Work out the finished part from the listing and answer in its coordinate system (mm). A direction names the side the tool comes from. Round coordinates to 2 decimals unless told otherwise and drop trailing zeros. Order: outer loops, then holes, each group sorted by start corner. A loop starts at its lowest first (then second) coordinate and runs counter-clockwise, first axis right, second up. Notation, with made-up numbers: M -21.5,54.25 L 14.5,54.25 A25 cw 14.5,89.25 Z; hole C -17,4 d1. An arc over 180 degrees is marked long. Return JSON: item names as keys, results as strings.
from build123d import *

# Parameters (mm, degrees)
SKETCH1_W           = 23
SKETCH1_H           = 30
SKETCH1_R           = 2.5
BOSS_EXTRUDE1_DEPTH = 6
BOSS_EXTRUDE2_START = -6
SKETCH2_R           = 4
BOSS_EXTRUDE2_DEPTH = 8


with BuildPart() as part:
    # Sketch1 → Boss-Extrude1 (new body)
    with BuildSketch(Plane(origin=(0, 0, 0), x_dir=(1, 0, 0), z_dir=(0, 1, 0))):
        Rectangle(SKETCH1_W, SKETCH1_H)
        with Locations((-8.4, 11.9)):
            Circle(SKETCH1_R, mode=Mode.SUBTRACT)
        with Locations((8.4, 11.9)):
            Circle(SKETCH1_R, mode=Mode.SUBTRACT)
    extrude(amount=BOSS_EXTRUDE1_DEPTH)

    # Sketch2 → Boss-Extrude2 (add)
    with BuildSketch(Plane(origin=(0, 6, 0), x_dir=(1, 0, 0), z_dir=(0, 1, 0)).offset(BOSS_EXTRUDE2_START)):
        Circle(SKETCH2_R)
    extrude(amount=BOSS_EXTRUDE2_DEPTH)


solid = part.part
Item 1: Find section A-A (z = -11.9). Determine the outline of the cut face in (x, y), plus the area to 3 significant figures.
Output:
{"outline": "M -11.5,0 L -10.9,0 L -10.9,6 L -11.5,6 Z; M -5.9,0 L 5.9,0 L 5.9,6 L -5.9,6 Z; M 10.9,0 L 11.5,0 L 11.5,6 L 10.9,6 Z", "area": "78.0 mm^2"}
Item 2: Each of these flat-tipped pins is pushed along its axis until it touches: pin 1 (6 mm diameter, centred on x = 7.5, z = 10.5, fed in from +Y); pin 2 (4 mm diameter, centred on x = -8.4, z = -11.9, fed in from -Y). Where does it stop, or does it pass through?
Output:
{"pin 1": "stops at y = 6", "pin 2": "passes through"}
Item 3: Find section C-C (y = 4.25). Determine the outline of the cut face in (x, z).
Output:
{"outline": "M -11.5,-15 L 11.5,-15 L 11.5,15 L -11.5,15 Z; hole C -8.4,-11.9 d5; hole C 8.4,-11.9 d5"}
Item 4: Consider line 1 along X through (y, z) = (1.8, -11.9); line 2 along Z through (x, y) = (-8.4, 3.5); line 3 along X through (y, z) = (5, -10.25). Determine where each line is inside the solid, lowest interval first. Write a range as [from, to].
Output:
{"line 1": "x = [-11.5, -10.9], [-5.9, 5.9], [10.9, 11.5]", "line 2": "z = [-15, -14.4], [-9.4, 15]", "line 3": "x = [-11.5, -10.28], [-6.52, 6.52], [10.28, 11.5]"}
Item 5: Find section D-D (x = 0). Determine the outline of the cut face in (y, z).
Output:
{"outline": "M 0,-15 L 6,-15 L 6,-4 L 8,-4 L 8,4 L 6,4 L 6,15 L 0,15 Z"}
Item 6: The mould has two halves that part along Z. Classify faces 1 (the flat face through (11.5, 3, 0)), 2 (the cylindrical face through (8.07, 2.96, -14.38)), 3 (the flat face through (0, 3, 15)): pulls with the +Z half, pulls with the -Z half, needs draft (parallel to the pull), parting line crosses it, or undercut.
Output:
{"face 1": "needs draft", "face 2": "undercut", "face 3": "pulls with the +Z half"}
Item 7: Which of the six approach directions +Z, -Z, +X, -X, +Y, -Y give full straight-line access (tool end or side, diameter ignored) to faces 4 (the flat face through (-3, 6, 3)), 5 (the cylindrical face through (-10.24, 2.96, -13.59))?
Output:
{"face 4": "+Y", "face 5": "+Y, -Y"}
Item 8: Find section B-B (x = 8.4). Determine the outline of the cut face in (y, z), plus the area to 3 significant figures.
Output:
{"outline": "M 0,-15 L 6,-15 L 6,-14.4 L 0,-14.4 Z; M 0,-9.4 L 6,-9.4 L 6,15 L 0,15 Z", "area": "150 mm^2"}
